```python
from build123d import *

# Parameters (mm, degrees)
SKETCH3_R                    = 15
SKETCH3_R_2                  = 10
BOSS_EXTRUDE1_DEPTH          = 10
SKETCH4_R                    = 2
CUT_EXTRUDE1_DEPTH           = 21
CUT_EXTRUDE1_TAPER           = 1
CUT_EXTRUDE1_OTHER_WAY_DEPTH = 19
CUT_EXTRUDE1_OTHER_WAY_TAPER = 1


with BuildPart() as part:
    # Sketch3 → Boss-Extrude1 (new body)
    with BuildSketch(Plane(origin=(0, 0, 0), x_dir=(1, 0, 0), z_dir=(0, 1, 0))):
        Circle(SKETCH3_R)
        Circle(SKETCH3_R_2, mode=Mode.SUBTRACT)
    extrude(amount=BOSS_EXTRUDE1_DEPTH)

    # Sketch4 → Cut-Extrude1 (cut)
    with BuildSketch(Plane.XY):
        with Locations((0, 5)):
            Circle(SKETCH4_R)
    extrude(amount=-CUT_EXTRUDE1_DEPTH, taper=CUT_EXTRUDE1_TAPER, mode=Mode.SUBTRACT)

    # Sketch4 → Cut-Extrude1 other way (cut)
    with BuildSketch(Plane.XY):
        with Locations((0, 5)):
            Circle(SKETCH4_R)
    extrude(amount=CUT_EXTRUDE1_OTHER_WAY_DEPTH, taper=CUT_EXTRUDE1_OTHER_WAY_TAPER, mode=Mode.SUBTRACT)


solid = part.part
```
Work out the finished part from the listing and answer in its coordinate system (mm). A direction names the side the tool comes from. Coordinates: 2 decimals unless noted, no trailing zeros. Loops run counter-clockwise (first coordinate to the right, second up) from the corner with the lowest first, then second, coordinate; pieces in that order, holes last. Notation, with made-up numbers: (73.5, 89.25) - (110.5, 89.25) arc R31 ccw to (110.5, 115.25) - close; hole circle Ø11 at (21.25, 88). An arc over 180 degrees is marked (long way). Use a Markdown table: item, result.
Item 1: The mould has two halves that part along Z. Classify faces 3 (the conical face through (-0.39, 3.26, -12.45)), 4 (the flat face through (3, 10, 10)), 5 (the cylindrical face through (-14.985, 4.93, -0.66)): +Z half, -Z half, draft (parallel to the pull), parting line (faces both ways), or undercut.
Evaluation:
| item | result |
|---|---|
| face 3 | undercut |
| face 4 | draft |
| face 5 | parting line |
Item 2: Find section C-C, the plane y = 9. Determine the outline of the cut face in (x, z), and give its area (3 significant figures).
Evaluation:
| item | result |
|---|---|
| outline | circle Ø30 at (0, 0); hole circle Ø20 at (0, 0) |
| area | 393 mm2 |
Item 3: Given pin 1 Ø4 at (y, z) = (8.5, -11.5) entering from -X; pin 2 Ø4 at (y, z) = (8.5, 9.5) entering from -X; pin 3 Ø3 at (y, z) = (2.5, 10.5) entering from -X, each flat-ended and moving along its own axis, determine where each tip first touches the part or whether it passes through.
Evaluation:
| item | result |
|---|---|
| pin 1 | stops at x = -11.61 |
| pin 2 | stops at x = -12.99 |
| pin 3 | stops at x = -12 |
Item 4: Find section A-A, the plane z = 0. Determine the outline of the cut face in (x, y), and give its area (3 significant figures).
Evaluation:
| item | result |
|---|---|
| outline | (-15, 0) - (-10, 0) - (-10, 10) - (-15, 10) - close; (10, 0) - (15, 0) - (15, 10) - (10, 10) - close |
| area | 100 mm2 |
Item 5: Consider probe 1 along X at (y, z) = (6, 0); probe 2 along X at (y, z) = (4.5, 1); probe 3 along Z at (x, y) = (-5, 1). Determine where each line is inside the solid, lowest interval first. Write a range as from..to.
Evaluation:
| item | result |
|---|---|
| probe 1 | x = -15..-10, 10..15 |
| probe 2 | x = -14.97..-9.95, 9.95..14.97 |
| probe 3 | z = -14.14..-8.66, 8.66..14.14 |
Item 6: For faces 1 (the conical face through (0.823, 3.418, 12.452)), 2 (the flat face through (3, 0, 10)), determine the directions among +Z, -Z, +X, -X, +Y, -Y from which every point of the face is accessible in a straight line to the end or side of a thin tool.
Evaluation:
| item | result |
|---|---|
| face 1 | none |
| face 2 | +Z, -Z, +X, -X, -Y |
Item 7: Find section B-B, the plane x = 6. Determine the outline of the cut face in (y, z), and give its area (3 significant figures).
Evaluation:
| item | result |
|---|---|
| outline | (0, -13.75) - (10, -13.75) - (10, -8) - (0, -8) - close; (0, 8) - (10, 8) - (10, 13.75) - (0, 13.75) - close |
| area | 115 mm2 |
Item 8: Find section D-D, the plane z = 11.5. Determine the outline of the cut face in (x, y), and give its area (3 significant figures).
Evaluation:
| item | result |
|---|---|
| outline | (-9.63, 0) - (9.63, 0) - (9.63, 10) - (-9.63, 10) - close; hole circle Ø3.6 at (0, 5) |
| area | 182 mm2 |
